Input: part model. Units: mm. Frame: model coordinates. Face numbers are marked on the shaded views. A direction names the side the tool comes from. Coordinates: 2 decimals unless noted, no trailing zeros. Write each loop counter-clockwise with the first axis right and the second up, starting at its lowest first coordinate (ties: lowest second). Pieces come first, ordered by that corner, then holes. Notation, with made-up numbers: M -13,24.5 L -3,24.5 A19 cw -3,59.5 Z; hole C 8.25,86 d5. An arc over 180 degrees is marked long. Use CSV: the item, a comma, the result in double quotes.
```python
from build123d import *

# Parameters (mm, degrees)
BOSS_EXTRUDE1_DEPTH = 13
SKETCH2_R           = 2.25
CUT_EXTRUDE1_DEPTH  = 65.730209331
SKETCH3_R           = 2
BOSS_EXTRUDE2_DEPTH = 3
BOSS_EXTRUDE3_START = 3
SKETCH4_R           = 2
BOSS_EXTRUDE3_DEPTH = 3
FILLET1_R           = 6.5
FILLET2_R           = 6.5


with BuildPart() as part:
    # Sketch1 → Boss-Extrude1 (new body)
    with BuildSketch(Plane.XY):
        Polygon((3, 0), (3, 32), (36, 32), (36, 0), (39, 0), (39, 36), (35.5, 36), (35.5, 50), (3.5, 50), (3.5, 36), (0, 36), (0, 0), align=None)
    extrude(amount=BOSS_EXTRUDE1_DEPTH)

    # Sketch2 → Cut-Extrude1 (cut, through all)
    with BuildSketch(Plane.ZY):
        with Locations((6.5, 5.293988539)):
            Circle(SKETCH2_R)
    extrude(amount=-CUT_EXTRUDE1_DEPTH, mode=Mode.SUBTRACT)

    # Sketch3 → Boss-Extrude2 (add)
    with BuildSketch(Plane.ZY.offset(-3.5)):
        with Locations(Location((6.5, 43.5, 0), (0, 0, 180))):
            Circle(SKETCH3_R)
    extrude(amount=BOSS_EXTRUDE2_DEPTH)

    # Sketch4 → Boss-Extrude3 (add)
    with BuildSketch(Plane(origin=(35.5, 0, 0), x_dir=(0, 0, -1), z_dir=(1, 0, 0)).offset(BOSS_EXTRUDE3_START)):
        with Locations((-6.5, 43.5)):
            Circle(SKETCH4_R)
    extrude(amount=-BOSS_EXTRUDE3_DEPTH)

    # Fillet1
    fillet1_edges = [part.edges().sort_by_distance(p)[0] for p in [
        (1.5, 0, 0),
        (1.5, 0, 13),
        (37.5, 0, 0),
        (37.5, 0, 13),
    ]]
    fillet(fillet1_edges, radius=FILLET1_R - 0.0001)  # a hair under: the kernel refuses the full size

    # Fillet2
    fillet2_edges = [part.edges().sort_by_distance(p)[0] for p in [
        (19.5, 50, 13),
        (19.5, 50, 0),
    ]]
    fillet(fillet2_edges, radius=FILLET2_R - 0.0001)  # a hair under: the kernel refuses the full size


solid = part.part
```
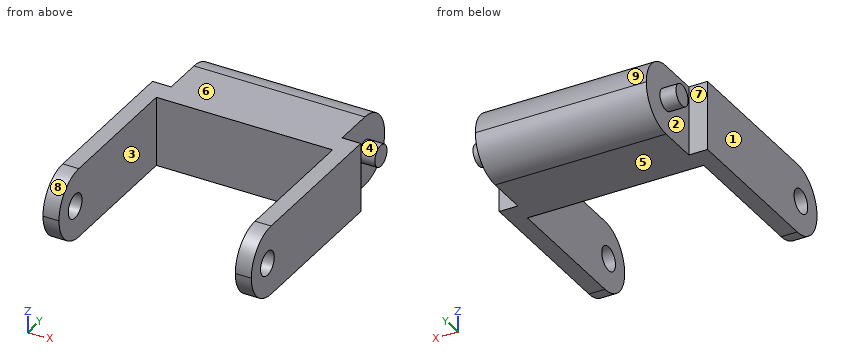
1. Contact query for flat-ended pins moving along their axis: pin 1 Ø1 at (x, z) = (1.5, 9.5) entering from +Y; pin 2 Ø5 at (x, z) = (14.5, 4.5) entering from +Y; pin 3 Ø4.5 at (y, z) = (43, 7.5) entering from +X; pin 4 Ø1 at (y, z) = (37.5, 6.5) entering from +X. Output: stop coordinate, or through.
Resolved:
pin 1,"stops at y = 36"
pin 2,"stops at y = 50"
pin 3,"stops at x = 38.5"
pin 4,"stops at x = 35.5"
2. Access query for the marked faces 1, 2, 3, 4 and 5. Directions: +Z, -Z, +X, -X, +Y, -Y. A direction counts if a zero-diameter tool reaches every point of the face in a straight line with its end or side. Return the directions, or none.
Resolved:
face 1,"+Z, -Z, -X, +Y, -Y"
face 2,"-X"
face 3,"+Z, -Z, -Y"
face 4,"+X"
face 5,"-Z, +X, -X, +Y, -Y"
3. Section D-D (y = 37). Return loops of the section in (x, z).
Resolved:
outline,"M 3.5,0 L 35.5,0 L 35.5,13 L 3.5,13 Z"
4. Mould query, pull axis Y, two halves, no side actions, for the marked faces 6, 7, 8 and 9. Classes: pulls with the +Y half, pulls with the -Y half, needs draft (parallel to the pull), parting line crosses it, or undercut.
Resolved:
face 6,"needs draft"
face 7,"undercut"
face 8,"pulls with the -Y half"
face 9,"pulls with the +Y half"
5. Section A-A (y = 28.5). Return loops of the section in (x, z).
Resolved:
outline,"M 0,0 L 3,0 L 3,13 L 0,13 Z; M 36,0 L 39,0 L 39,13 L 36,13 Z"
6. Section B-B (z = 11.5). Return loops of the section in (x, y), then the cut area to 3 significant figures.
Resolved:
outline,"M 0,2.35 L 3,2.35 L 3,32 L 36,32 L 36,2.35 L 39,2.35 L 39,36 L 35.5,36 L 35.5,47.65 L 3.5,47.65 L 3.5,36 L 0,36 Z"
area,"707 mm^2"
7. Material intervals for line 1 (Y direction, x = 37.6, z = 6.5); line 2 (X direction, y = 17, z = 5.25); line 3 (X direction, y = 37, z = 2.5), sorted ascending. Write a range as [from, to].
Resolved:
line 1,"y = [0, 3.04], [7.54, 36], [41.5, 45.5]"
line 2,"x = [0, 3], [36, 39]"
line 3,"x = [3.5, 35.5]"
